from build123d import *

# Parameters (mm, degrees)
F0_W     = 160
F0_H     = 170
F0_W_2   = 145
F0_H_2   = 135
F1_DEPTH = 3
F2_W     = 147
F2_H     = 137
F2_W_2   = 145
F2_H_2   = 135
F3_DEPTH = 65
F4_W     = 147
F4_H     = 137
F5_DEPTH = 1


with BuildPart() as f1:
    # F0 (on Top) → F1 (new body)
    with BuildSketch(Plane.XY):
        Rectangle(F0_W, F0_H)
        Rectangle(F0_W_2, F0_H_2, mode=Mode.SUBTRACT)
    extrude(amount=-F1_DEPTH)

    # F2 (on face) → F3 (join)
    with BuildSketch(Plane(origin=(0, 0, -3), x_dir=(1, 0, 0), z_dir=(0, 0, -1))):
        Rectangle(F2_W, F2_H)
        Rectangle(F2_W_2, F2_H_2, mode=Mode.SUBTRACT)
    extrude(amount=F3_DEPTH)

    # F4 (on face) → F5 (join)
    with BuildSketch(Plane(origin=(0, 0, -68), x_dir=(1, 0, 0), z_dir=(0, 0, -1))):
        Rectangle(F4_W, F4_H)
    extrude(amount=F5_DEPTH)


solid = f1.part
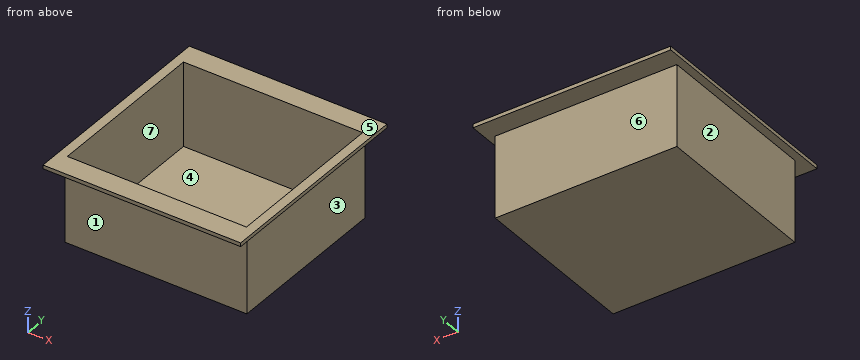
Work out the finished part from the listing and answer in its coordinate system (mm). Face numbers are marked on the shaded views. A direction names the side the tool comes from. Round coordinates to 2 decimals unless told otherwise and drop trailing zeros. Order: outer loops, then holes, each group sorted by start corner. A loop starts at its lowest first (then second) coordinate and runs counter-clockwise, first axis right, second up. Notation, with made-up numbers: M 64.5,35 L 103.5,35 A30 ccw 103.5,61 Z; hole C 71.5,4 d1. An arc over 180 degrees is marked long. Put each result on its own line as item: value. Start each with the question number.
Q1. Section C-C, the plane y = 35 is taken. Write down the section's boundary in (x, z), and give its area (3 significant figures).
Q2. For a pull along X with two mould halves and no side action, classify the marked faces 1, 2, 3 and 4 as pulls with the +X half, pulls with the -X half, needs draft (parallel to the pull), parting line crosses it, or undercut.
Q3. Flat-ended cylindrical pins translate along their axes: pin 1 (8 mm diameter, centred on x = 25, z = -37.5, fed in from -Y); pin 2 (3 mm diameter, centred on x = 48.5, y = -16.5, fed in from +Z); pin 3 (6 mm diameter, centred on y = 7, z = -55.5, fed in from +X). Find the tip coordinate at first contact, or state that the pin passes through.
Q4. A tool of negligible diameter and unlimited length cuts with its end or side. For the marked faces 5, 6 and 7, from which of +Z, -Z, +X, -X, +Y, -Y can it reach the whole face along a straight path? Write none if from no direction.
Q5. Section B-B, the plane x = -57.5 is taken. Write down the section's boundary in (y, z).
Q6. Straight lines are drawn through the part: L1, parallel to X at y = 0, z = -5; L2, parallel to Y at x = 48.5, z = -56; L3, parallel to Z at x = -70.5, y = 60. For each, find the intervals that lie inside material, in ascending order. Write a range as [from, to].
Q7. Section A-A, the plane z = -58 is taken. Write down the section's boundary in (x, y).
Findings below:
1. outline: M -80,-3 L -73.5,-3 L -73.5,-69 L 73.5,-69 L 73.5,-3 L 80,-3 L 80,0 L 72.5,0 L 72.5,-68 L -72.5,-68 L -72.5,0 L -80,0 Z
1. area: 322 mm^2
2. face 1: needs draft
2. face 2: pulls with the -X half
2. face 3: pulls with the +X half
2. face 4: undercut
3. pin 1: stops at y = -68.5
3. pin 2: stops at z = -68
3. pin 3: stops at x = 73.5
4. face 5: +Z, +X, -X, +Y, -Y
4. face 6: -Z, +X, -X, +Y
4. face 7: +Z
5. outline: M -85,-3 L -68.5,-3 L -68.5,-69 L 68.5,-69 L 68.5,-3 L 85,-3 L 85,0 L 67.5,0 L 67.5,-68 L -67.5,-68 L -67.5,0 L -85,0 Z
6. L1: x = [-73.5, -72.5], [72.5, 73.5]
6. L2: y = [-68.5, -67.5], [67.5, 68.5]
6. L3: z = [-69, -68]
7. outline: M -73.5,-68.5 L 73.5,-68.5 L 73.5,68.5 L -73.5,68.5 Z; hole M -72.5,-67.5 L 72.5,-67.5 L 72.5,67.5 L -72.5,67.5 Z
